For this review, take the finished solid that the model builds, in its own axes (mm). A direction names the side the tool comes from. Coordinates: 2 decimals unless noted, no trailing zeros. Loops run counter-clockwise (first coordinate to the right, second up) from the corner with the lowest first, then second, coordinate; pieces in that order, holes last.
1. Take a section at A-A, the plane y = -12. State the section outline as (x, z) points.
2. To check wall thickness, follow probe 1 along Y at (x, z) = (-18, 3.6); probe 2 along X at (y, z) = (12, 0.5); probe 3 along X at (y, z) = (17, 1.25). State the ranges of each line that lie inside material, in increasing order.
3. Clearance check with flat-ended pins moving along their axes: P1, Ø1.2, axis at x = -1.5, z = 2.5, coming from the -Y side; P2, Ø1.2, axis at x = 1, z = 1, coming from the +Y side; P3, Ø1, axis at x = 4, z = 3, coming from the -Y side. State where each tip first meets the part, or that it passes through.
4. Mouldability with a two-part tool opening along X and no side actions: class faces 4 (the face through (23.74, -5.22, 2.03)), 5 (the face through (33.187, -22.33, 1.972)), 6 (the face through (0.6, -8.3, 4)), 7 (the face through (-27.24, -26.66, 1.97)) as pulls with the +X half, pulls with the -X half, needs draft (parallel to the pull), parting line crosses it, or undercut.
5. Machinability: for faces 1 (the face through (18.48, 10.79, 2.03)), 2 (the face through (-26.66, 27.24, 1.97)), 3 (the face through (-35.091, 14.593, 1.972)), which of the approach directions +Z, -Z, +X, -X, +Y, -Y give a long, thin tool a straight path to every point of the face, cutting with its end or side? Answer none if there is none.
6. Take a section at B-B, the plane y = 3. State the section outline as (x, z) points, then the cut area to 3 significant figures.
7. Take a section at C-C, the plane x = -35. State the section outline as (y, z) points, then the cut area to 3 significant figures.
8. Take a section at D-D, the plane z = 2.25. Count the separate pieces of the cut face and the enclosed holes in it, then the cut area to 3 significant figures.
```python
from build123d import *

# Parameters (mm, degrees)
AUFSATZ_LINEAR_AUSTRAGEN1_DEPTH = 4
SCHNITT_LINEAR_AUSTRAGEN1_REACH = 6
SKIZZE2_R                       = 8
SKIZZE4_W                       = 14.7
SKIZZE4_H                       = 3.6
SCHNITT_LINEAR_AUSTRAGEN2_DEPTH = 4
KREISMUSTER1_COUNT              = 6
SKIZZE5_R                       = 0.5
SCHNITT_LINEAR_AUSTRAGEN3_DEPTH = 4
KREISMUSTER2_COUNT              = 3


with BuildPart() as part:
    # Skizze1 → Aufsatz-Linear austragen1 (new body)
    with BuildSketch(Plane.XY):
        with BuildLine():
            Line((0, 36.168934028), (14.18455057, 33.162270875))
            Line((14.18455057, 33.162270875), (15.013991658, 37.075329459))
            ThreePointArc((15.013991658, 37.075329459), (22.427500118, 33.121099596), (28.851450623, 27.705483157))
            Line((28.851450623, 27.705483157), (25.57529852, 25.57529852))
            Line((25.57529852, 25.57529852), (33.479258511, 13.41927472))
            Line((33.479258511, 13.41927472), (36.832712189, 15.599721561))
            ThreePointArc((36.832712189, 15.599721561), (39.278791543, 7.561516706), (39.991791399, -0.810321366))
            Line((39.991791399, -0.810321366), (36.168934028, 0))
            Line((36.168934028, 0), (33.162270875, -14.18455057))
            Line((33.162270875, -14.18455057), (37.075329459, -15.013991658))
            ThreePointArc((37.075329459, -15.013991658), (33.121099596, -22.427500118), (27.705483157, -28.851450623))
            Line((27.705483157, -28.851450623), (25.57529852, -25.57529852))
            Line((25.57529852, -25.57529852), (13.41927472, -33.479258511))
            Line((13.41927472, -33.479258511), (15.599721561, -36.832712189))
            ThreePointArc((15.599721561, -36.832712189), (7.561516706, -39.278791543), (-0.810321366, -39.991791399))
            Line((-0.810321366, -39.991791399), (0, -36.168934028))
            Line((0, -36.168934028), (-14.18455057, -33.162270875))
            Line((-14.18455057, -33.162270875), (-15.013991658, -37.075329459))
            ThreePointArc((-15.013991658, -37.075329459), (-22.427500118, -33.121099596), (-28.851450623, -27.705483157))
            Line((-28.851450623, -27.705483157), (-25.57529852, -25.57529852))
            Line((-25.57529852, -25.57529852), (-33.479258511, -13.41927472))
            Line((-33.479258511, -13.41927472), (-36.832712189, -15.599721561))
            ThreePointArc((-36.832712189, -15.599721561), (-39.278791543, -7.561516706), (-39.991791399, 0.810321366))
            Line((-39.991791399, 0.810321366), (-36.168934028, 0))
            Line((-36.168934028, 0), (-33.162270875, 14.18455057))
            Line((-33.162270875, 14.18455057), (-37.075329459, 15.013991658))
            ThreePointArc((-37.075329459, 15.013991658), (-33.121099596, 22.427500118), (-27.705483157, 28.851450623))
            Line((-27.705483157, 28.851450623), (-25.57529852, 25.57529852))
            Line((-25.57529852, 25.57529852), (-13.41927472, 33.479258511))
            Line((-13.41927472, 33.479258511), (-15.599721561, 36.832712189))
            ThreePointArc((-15.599721561, 36.832712189), (-7.561516706, 39.278791543), (0.810321366, 39.991791399))
            Line((0.810321366, 39.991791399), (0, 36.168934028))
        make_face()
    extrude(amount=AUFSATZ_LINEAR_AUSTRAGEN1_DEPTH)

    # Skizze2 → Schnitt-Linear austragen1 (cut, up to next)
    with BuildSketch(Plane.XY.offset(4), mode=Mode.PRIVATE) as schnitt_linear_austragen1_sk1:
        Circle(SKIZZE2_R)
    schnitt_linear_austragen1_tool1 = extrude(schnitt_linear_austragen1_sk1.sketch, amount=-SCHNITT_LINEAR_AUSTRAGEN1_REACH, mode=Mode.PRIVATE) & part.part
    add(schnitt_linear_austragen1_tool1.solids().sort_by_distance((0, 0, 4))[0], mode=Mode.SUBTRACT)

    # Skizze4 → Schnitt-Linear austragen2 (cut)
    with BuildSketch(Plane.XY.offset(4)):
        with Locations((0, 23.2)):
            Rectangle(SKIZZE4_W, SKIZZE4_H)
    schnitt_linear_austragen2 = extrude(amount=-SCHNITT_LINEAR_AUSTRAGEN2_DEPTH, mode=Mode.SUBTRACT)

    # Kreismuster1: Schnitt-Linear austragen2 ×6 about axis
    kreismuster1_axis = Axis((0, 0, 0), (0, 0, 1))
    for i in range(1, KREISMUSTER1_COUNT):
        add(schnitt_linear_austragen2.rotate(kreismuster1_axis, i * 360 / KREISMUSTER1_COUNT), mode=Mode.SUBTRACT)

    # Skizze5 → Schnitt-Linear austragen3 (cut)
    with BuildSketch(Plane.XY.offset(4)):
        with Locations((0, 31)):
            Circle(SKIZZE5_R)
    schnitt_linear_austragen3 = extrude(amount=-SCHNITT_LINEAR_AUSTRAGEN3_DEPTH, mode=Mode.SUBTRACT)

    # Kreismuster2: Schnitt-Linear austragen3 ×3 about axis
    kreismuster2_axis = Axis((0, 0, 0), (0, 0, 1))
    for i in range(1, KREISMUSTER2_COUNT):
        add(schnitt_linear_austragen3.rotate(kreismuster2_axis, i * 360 / KREISMUSTER2_COUNT), mode=Mode.SUBTRACT)


solid = part.part
```
Results list:
1. outline: (-38.16, 0) - (-21.94, 0) - (-21.94, 4) - (-38.16, 4) - close; (-17.78, 0) - (17.78, 0) - (17.78, 4) - (-17.78, 4) - close; (21.94, 0) - (33.63, 0) - (33.63, 4) - (21.94, 4) - close
2. probe 1: y = -35.72 to -18.82, -11.62 to 11.62, 18.82 to 30.5
2. probe 2: x = -33.63 to -21.94, -17.78 to 17.78, 21.94 to 38.16
2. probe 3: x = -36.21 to -19.05, -14.9 to 14.9, 19.05 to 31.15
3. P1: stops at y = -35.98
3. P2: stops at y = 40
3. P3: stops at y = -39.85
4. face 4: undercut
4. face 5: pulls with the +X half
4. face 6: needs draft
4. face 7: pulls with the -X half
5. face 1: +Z, -Z
5. face 2: +Z, -Z, +Y
5. face 3: +Z, -Z, -X
6. outline: (-35.53, 0) - (-7.42, 0) - (-7.42, 4) - (-35.53, 4) - close; (7.42, 0) - (39.89, 0) - (39.89, 4) - (7.42, 4) - close
6. area: 242 mm2
7. outline: (-14.41, 0) - (5.51, 0) - (5.51, 4) - (-14.41, 4) - close; (14.57, 0) - (19.36, 0) - (19.36, 4) - (14.57, 4) - close
7. area: 98.9 mm2
8. separate pieces: 1
8. enclosed holes: 10
8. area: 4,000 mm2
